Autodesk Inventor part; units mm, degrees
ref_plane "YZ Plane" through (0, 0, 0) normal (1, 0, 0) x (0, 1, 0)
ref_plane "XZ Plane" through (0, 0, 0) normal (0, 1, 0) x (-1, 0, 0)
ref_plane "XY Plane" through (0, 0, 0) normal (0, 0, 1) x (1, 0, 0)
sketch "Sketch1" plane through (0, 0, 0) normal (0, 1, 0) x (-1, 0, 0)
  line L0 (8, 0) -> (102.94, 0)
  line L1 (110.94, -8) -> (110.94, -185.2)
  line L2 (102.94, -193.2) -> (8, -193.2)
  line L3 (0, -185.2) -> (0, -8)
  circle A0 centre (86.7029, -32) radius 2.1
  circle A1 centre (88.297, -158.2) radius 2.1
  circle A2 centre (22.6, -158.501) radius 2.1
  circle A3 centre (21.4029, -32) radius 2.1
  arc A4 (110.94, -8) -> (102.94, 0) centre (102.94, -8) ccw
  arc A5 (8, 0) -> (0, -8) centre (8, -8) ccw
  arc A6 (0, -185.2) -> (8, -193.2) centre (8, -185.2) ccw
  arc A7 (102.94, -193.2) -> (110.94, -185.2) centre (102.94, -185.2) ccw
  point P0 (0, 0)
  dimension "d0" = 110.94
  dimension "d1" = 193.2
  dimension "d2" = 4.2
  dimension "d3" = 4.2
  dimension "d4" = 65.3
  dimension "d5" = 65.697
  dimension "d6" = 4.2
  dimension "d7" = 4.2
  dimension "d8" = 126.2
  dimension "d9" = 126.501
  dimension "d10" = 0
  dimension "d11" = 22.6
  dimension "d12" = 35
  dimension "d13" = 8
extrude "Extrusion1" add sketch "Sketch1" along normal blind 2
sketch "Sketch2" plane through (0, 2, 0) normal (0, 1, 0) x (1, 0, 0)
  line L0 (-8, 193.2) -> (-102.94, 193.2)
  arc A0 (-102.94, 193.2) -> (-110.94, 185.2) centre (-102.94, 185.2) ccw
  line L1 (-110.94, 185.2) -> (-110.94, 8)
  arc A1 (-110.94, 8) -> (-102.94, 0) centre (-102.94, 8) ccw
  line L2 (-102.94, 0) -> (-8, 0)
  arc A2 (-8, 0) -> (0, 8) centre (-8, 8) ccw
  line L3 (0, 8) -> (0, 185.2)
  arc A3 (0, 185.2) -> (-8, 193.2) centre (-8, 185.2) ccw
  circle A4 centre (-86.7029, 32) radius 2.1
  circle A5 centre (-88.297, 158.2) radius 2.1
  circle A6 centre (-22.6, 158.501) radius 2.1
  circle A7 centre (-21.4029, 32) radius 2.1
  line L4 (-108.94, 11) -> (-108.94, 179.2)
  line L5 (-108.94, 179.2) -> (-6, 179.2)
  line L6 (-6, 11) -> (-108.94, 11)
  line L7 (-6, 179.2) -> (-6, 11)
  point P0 (0, 0)
  dimension "d16" = 2
  dimension "d17" = 14
  dimension "d18" = 11
  dimension "d19" = 6
extrude "Extrusion2" add sketch "Sketch2" along normal blind 7.5 contours A3 L3 A2 L2 A1 L1 A0 L0
sketch "Sketch3" plane through (0, 2, 0) normal (0, 1, 0) x (1, 0, 0)
  line L0 (-91, 41) -> (-12, 41)
  line L1 (-12, 41) -> (-12, 146)
  line L2 (-12, 146) -> (-91, 146)
  line L3 (-6, 179.2) -> (-6, 11)
  line L4 (-6, 11) -> (-108.94, 11)
  line L5 (-99.94, 72) -> (-91, 72)
  line L6 (-91, 118.2) -> (-99.94, 118.2)
  line L7 (-99.94, 118.2) -> (-99.94, 72)
  circle A0 centre (-88.297, 158.2) radius 2.1
  circle A1 centre (-86.7029, 32) radius 2.1
  line L8 (-108.94, 11) -> (-108.94, 179.2)
  line L9 (-91, 146) -> (-91, 118.2)
  line L10 (-91, 72) -> (-91, 41)
  point P0 (0, 0)
  dimension "d22" = 105
  dimension "d24" = 6
  dimension "d25" = 30
  dimension "d26" = 40
  dimension "d27" = 40
  dimension "d28" = 9
extrude "Extrusion3" cut sketch "Sketch3" against normal blind 7.5 contours L10 L5 L7 L6 L9 L2 L1 L0
properties part number "Front"
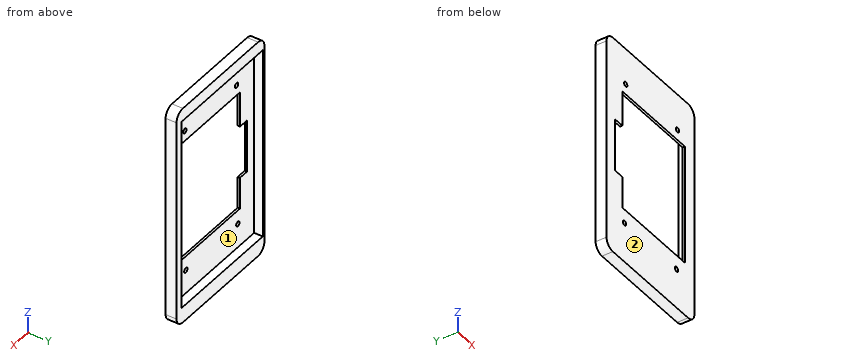
Could you check a few things on this model? Use its own coordinates, in mm. Face numbers are marked on the shaded views. Round coordinates to 2 decimals unless told otherwise and drop trailing zeros. Loops run counter-clockwise (first coordinate to the right, second up) from the corner with the lowest first, then second, coordinate; pieces in that order, holes last.
Q1. Thinking about a two-plate mould opening in Z: for the marked faces 1 and 2, which applies, pulls with the +Z half, pulls with the -Z half, needs draft (parallel to the pull), parting line crosses it, or undercut?
Q2. I want a section at A-A (z = -125). Write out the boundary of the cut face in (x, y), and give its area (3 significant figures).
Q3. I want a section at C-C (y = 5). Write out the boundary of the cut face in (x, z), and give its area (3 significant figures).
Q4. I want a section at B-B (x = -61.5). Write out the boundary of the cut face in (y, z), and give its area (3 significant figures).
Q5. For P1, Ø6, axis at x = -72, z = -171, coming from the +Y side; P2, Ø4, axis at x = -22.6, z = -158.501, coming from the +Y side, each with a flat end and sliding along its axis, tell me the tip position at first contact or that it passes through.
Q6. Please list where these lines run through material, in increasing order: L1, parallel to X at y = 1, z = -158.2; L2, parallel to Z at x = -37.5, y = 1.5; L3, parallel to X at y = 5.5, z = -156.
Q7. I want a section at D-D (z = -32). Write out the boundary of the cut face in (x, y), and give its area (3 significant figures).
Answer below:
1. face 1: undercut
1. face 2: needs draft
2. outline: (-110.94, 0) - (-91, 0) - (-91, 2) - (-108.94, 2) - (-108.94, 9.5) - (-110.94, 9.5) - close; (-12, 0) - (0, 0) - (0, 9.5) - (-6, 9.5) - (-6, 2) - (-12, 2) - close
2. area: 124 mm2
3. outline: (-110.94, -185.2) arc R8 ccw to (-102.94, -193.2) - (-8, -193.2) arc R8 ccw to (0, -185.2) - (0, -8) arc R8 ccw to (-8, 0) - (-102.94, 0) arc R8 ccw to (-110.94, -8) - close; hole (-108.94, -179.2) - (-6, -179.2) - (-6, -11) - (-108.94, -11) - close
3. area: 4,060 mm2
4. outline: (0, -193.2) - (9.5, -193.2) - (9.5, -179.2) - (2, -179.2) - (2, -146) - (0, -146) - close; (0, -41) - (2, -41) - (2, -11) - (9.5, -11) - (9.5, 0) - (0, 0) - close
4. area: 364 mm2
5. P1: stops at y = 2
5. P2: passes through
6. L1: x = -110.94 to -90.4, -86.2 to -24.68, -20.52 to 0
6. L2: z = -193.2 to -146, -41 to 0
6. L3: x = -110.94 to -108.94, -6 to 0
7. outline: (-110.94, 0) - (-88.8, 0) - (-88.8, 2) - (-108.94, 2) - (-108.94, 9.5) - (-110.94, 9.5) - close; (-84.6, 0) - (-23.5, 0) - (-23.5, 2) - (-84.6, 2) - close; (-19.3, 0) - (0, 0) - (0, 9.5) - (-6, 9.5) - (-6, 2) - (-19.3, 2) - close
7. area: 265 mm2
